Source: CAD feature listing. Evaluate the final solid. Frame: model axes, mm. Give positions to 0.01 mm unless a question says otherwise; leave off trailing zeros. Order: outer loops, then holes, each group sorted by start corner. A loop starts at its lowest first (then second) coordinate and runs counter-clockwise, first axis right, second up. Notation, with made-up numbers: (37.5, 79) -> (55.5, 79) arc R12 ccw to (55.5, 91) -> close; hole circle Ø8 at (-13, -3.75). An arc over 180 degrees is marked (long way). Use CSV: the item, a comma, the result in double quotes.
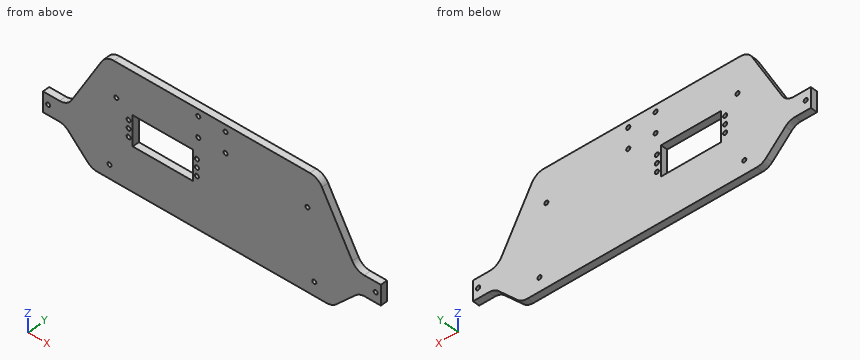
```python
from build123d import *

# Parameters (mm, degrees)
SALIENTE_EXTRUIR1_DEPTH = 5
REDONDEO1_R             = 10
CROQUIS2_R              = 1.5
CROQUIS2_W              = 42
CROQUIS2_H              = 20
CORTAR_EXTRUIR1_DEPTH   = 135.669558943
CROQUIS3_W              = 4
CROQUIS3_H              = 14.636342218
CORTAR_EXTRUIR2_DEPTH   = 135.669558943
CROQUIS4_W              = 44
CROQUIS4_H              = 22
CORTAR_EXTRUIR3_DEPTH   = 131.881206084


with BuildPart() as part:
    # Croquis1 → Saliente-Extruir1 (new body)
    with BuildSketch(Plane(origin=(0, 0, 0), x_dir=(1, 0, 0), z_dir=(0, 1, 0))):
        Polygon((-88.1, 42.318171109), (88.1, 42.318171109), (108.1, 22.318171109), (127.75, 22.318171109), (127.75, 7.681828891), (105.75, 7.681828891), (77.75, -42.318171109), (-77.75, -42.318171109), (-105.75, 7.681828891), (-127.75, 7.681828891), (-127.75, 22.318171109), (-108.1, 22.318171109), align=None)
    extrude(amount=SALIENTE_EXTRUIR1_DEPTH)

    # Redondeo1
    redondeo1_edges = [part.edges().sort_by_distance(p)[0] for p in [
        (-88.1, 2.5, -42.318171109),
        (88.1, 2.5, -42.318171109),
        (108.1, 2.5, -22.318171109),
        (105.75, 2.5, -7.681828891),
        (77.75, 2.5, 42.318171109),
        (-77.75, 2.5, 42.318171109),
        (-105.75, 2.5, -7.681828891),
        (-108.1, 2.5, -22.318171109),
    ]]
    fillet(redondeo1_edges, radius=REDONDEO1_R)

    # Croquis2 → Cortar-Extruir1 (cut, through all)
    with BuildSketch(Plane(origin=(0, 5, 0), x_dir=(1, 0, 0), z_dir=(0, 1, 0))):
        with Locations(Location((70, -17.318171109, 0), (0, 0, 270))):
            Circle(CROQUIS2_R)
        with Locations(Location((-70, -17.318171109, 0), (0, 0, 270))):
            Circle(CROQUIS2_R)
        with Locations(Location((-119.996067812, 15, 0), (0, 0, 270))):
            Circle(CROQUIS2_R)
        with Locations(Location((119.996067812, 15, 0), (0, 0, 270))):
            Circle(CROQUIS2_R)
        with Locations(Location((-75, 32.318171109, 0), (0, 0, 270))):
            Circle(CROQUIS2_R)
        with Locations(Location((75, 32.318171109, 0), (0, 0, 270))):
            Circle(CROQUIS2_R)
        with Locations(Location((-10, -22.318171109, 0), (0, 0, 270))):
            Circle(CROQUIS2_R)
        with Locations(Location((10, -22.318171109, 0), (0, 0, 270))):
            Circle(CROQUIS2_R)
        with Locations(Location((-10, -37.318171109, 0), (0, 0, 270))):
            Circle(CROQUIS2_R)
        with Locations(Location((10, -37.318171109, 0), (0, 0, 270))):
            Circle(CROQUIS2_R)
        with Locations(Location((-61, -0.681828891, 0), (0, 0, 270))):
            Circle(CROQUIS2_R)
        with Locations(Location((-11, -0.681828891, 0), (0, 0, 270))):
            Circle(CROQUIS2_R)
        with Locations(Location((-61, 5.318171109, 0), (0, 0, 270))):
            Circle(CROQUIS2_R)
        with Locations(Location((-61, -6.681828891, 0), (0, 0, 270))):
            Circle(CROQUIS2_R)
        with Locations(Location((-11, 5.318171109, 0), (0, 0, 270))):
            Circle(CROQUIS2_R)
        with Locations(Location((-11, -6.681828891, 0), (0, 0, 270))):
            Circle(CROQUIS2_R)
        with Locations((-36, -0.681828891)):
            Rectangle(CROQUIS2_W, CROQUIS2_H)
    extrude(amount=-CORTAR_EXTRUIR1_DEPTH, mode=Mode.SUBTRACT)

    # Croquis3 → Cortar-Extruir2 (cut, through all)
    with BuildSketch(Plane(origin=(0, 5, 0), x_dir=(1, 0, 0), z_dir=(0, 1, 0))):
        with Locations((-125.75, 15)):
            Rectangle(CROQUIS3_W, CROQUIS3_H)
        with Locations((125.75, 15)):
            Rectangle(CROQUIS3_W, CROQUIS3_H)
    extrude(amount=-CORTAR_EXTRUIR2_DEPTH, mode=Mode.SUBTRACT)

    # Croquis4 → Cortar-Extruir3 (cut, through all)
    with BuildSketch(Plane(origin=(0, 5, 0), x_dir=(1, 0, 0), z_dir=(0, 1, 0))):
        with Locations((-36, -0.681828891)):
            Rectangle(CROQUIS4_W, CROQUIS4_H)
    extrude(amount=-CORTAR_EXTRUIR3_DEPTH, mode=Mode.SUBTRACT)


solid = part.part
```
1. Pin query (flat end, axial travel): P1, Ø1.5, axis at y = 2.5, z = -2.5, coming from the +X side; P2, Ø1, axis at y = 2, z = -27.5, coming from the -X side; P3, Ø1.5, axis at y = 2, z = 4, coming from the -X side. Return the tip coordinate at first contact, or that it passes through.
Answer below:
P1,"stops at x = 103.3"
P2,"stops at x = -103.42"
P3,"stops at x = -99.63"
2. Section query B-B on z = 28. Return loops of the section in (x, y).
Answer below:
outline,"(-85.77, 0) -> (85.77, 0) -> (85.77, 5) -> (-85.77, 5) -> close"
3. Section query C-C on y = 0.85. Count the separate pieces of the cut face and the enclosed holes in it, plus the area to 3 significant figures.
Answer below:
separate pieces,"1"
enclosed holes,"17"
area,"15,600 mm²"
4. Section query A-A on x = -21. Return loops of the section in (y, z), plus the area to 3 significant figures.
Answer below:
outline,"(0, -42.32) -> (5, -42.32) -> (5, -10.32) -> (0, -10.32) -> close; (0, 11.68) -> (5, 11.68) -> (5, 42.32) -> (0, 42.32) -> close"
area,"313 mm²"
5. Ray query, line 1 along X through (y, z) = (1.9, 2); line 2 along Z through (x, y) = (-70, 2.2); line 3 along Z through (x, y) = (-16, 3.1). Return the intervals inside material, ascending.
Answer below:
line 1,"x = -100.33 to -61.72, -60.28 to -58, -14 to -11.72, -10.28 to 100.33"
line 2,"z = -42.32 to 15.82, 18.82 to 42.32"
line 3,"z = -42.32 to -10.32, 11.68 to 42.32"
